from build123d import *
from OCP.BRepFilletAPI import BRepFilletAPI_MakeChamfer

# Parameters (mm, degrees)
BOSS_EXTRUDE1_DEPTH = 30
CUT_EXTRUDE1_REACH  = 253.063
SKETCH10_W          = 41.5
SKETCH10_H          = 34
BOSS_EXTRUDE3_DEPTH = 4
CHAMFER4_SIZE       = 20
CHAMFER4_SIZE2      = 11.547005384
SKETCH11_W          = 20.75
SKETCH11_H          = 166.64
BOSS_EXTRUDE4_DEPTH = 4
SKETCH12_W          = 20.75
SKETCH12_H          = 18.32
BOSS_EXTRUDE5_DEPTH = 4
SKETCH13_W          = 75
SKETCH13_H          = 20
SKETCH13_W_2        = 20
SKETCH13_H_2        = 90
CUT_EXTRUDE2_DEPTH  = 4
FILLET1_R           = 3
CUT_EXTRUDE3_REACH  = 188.866
SKETCH15_R          = 1.6
CUT_EXTRUDE4_START  = -2
SKETCH16_R          = 3.5
SKETCH16_R_2        = 1.6
CUT_EXTRUDE4_DEPTH  = 2


with BuildPart() as part:
    # Sketch6 → Boss-Extrude1 (new body)
    with BuildSketch(Plane(origin=(0, 0, 0), x_dir=(1, 0, 0), z_dir=(0, 1, 0))):
        Polygon((0, -87.32), (37.5, -87.32), (37.5, -117.32), (90.67, -117.32), (142.319755082, -87.5), (142.319755082, 87.5), (90.67, 117.32), (37.5, 117.32), (37.5, 87.32), (0, 87.32), (0, 83.32), (41.5, 83.32), (41.5, 113.32), (89.59820323, 113.32), (138.319755082, 85.190598923), (138.319755082, -85.190598923), (89.59820323, -113.32), (41.5, -113.32), (41.5, -83.32), (0, -83.32), align=None)
    extrude(amount=BOSS_EXTRUDE1_DEPTH)

    # Sketch9 → Cut-Extrude1 (cut, up to next)
    with BuildSketch(Plane.XY.offset(87.32), mode=Mode.PRIVATE) as cut_extrude1_sk1:
        Polygon((37.5, 0), (15, 8), (0, 8), (0, 0), align=None)
    cut_extrude1_tool1 = extrude(cut_extrude1_sk1.sketch, amount=-CUT_EXTRUDE1_REACH, mode=Mode.PRIVATE) & part.part
    cut_extrude1 = cut_extrude1_tool1.solids().sort_by_distance((13.928571, 3.428571, 87.32))[0]
    add(cut_extrude1, mode=Mode.SUBTRACT)

    # Sketch10 → Boss-Extrude3 (add)
    with BuildSketch(Plane(origin=(0, 30, 0), x_dir=(1, 0, 0), z_dir=(0, 1, 0))):
        with Locations((20.75, -100.32)):
            Rectangle(SKETCH10_W, SKETCH10_H)
    boss_extrude3 = extrude(amount=-BOSS_EXTRUDE3_DEPTH)

    # Mirror1: Cut-Extrude1, Boss-Extrude3 across plane
    add(cut_extrude1.mirror(Plane.XY), mode=Mode.SUBTRACT)
    add(boss_extrude3.mirror(Plane.XY))

    # Chamfer4: one chamfer whose edges measure the first distance from different faces: ONE call of the kernel's chamfer builder (chamfer() names one face for all edges)
    chamfer4_edges_1 = [part.edges().sort_by_distance(p)[0] for p in [
        (37.5, 26, -102.32),
    ]]
    chamfer4_side_1 = [part.faces().sort_by_distance(p)[0] for p in [
        (18.75, 26, -102.32),
    ]]
    chamfer4_edges_2 = [part.edges().sort_by_distance(p)[0] for p in [
        (37.5, 26, 102.32),
    ]]
    chamfer4_side_2 = [part.faces().sort_by_distance(p)[0] for p in [
        (18.75, 26, 102.32),
    ]]
    chamfer4 = BRepFilletAPI_MakeChamfer(part.part.solid().wrapped)
    for e in chamfer4_edges_1:
        chamfer4.Add(CHAMFER4_SIZE, CHAMFER4_SIZE2, e.wrapped, chamfer4_side_1[0].wrapped)  # the first distance lies on this face
    for e in chamfer4_edges_2:
        chamfer4.Add(CHAMFER4_SIZE, CHAMFER4_SIZE2, e.wrapped, chamfer4_side_2[0].wrapped)  # the first distance lies on this face
    add(Compound.cast(chamfer4.Shape()), mode=Mode.REPLACE)

    # Sketch11 → Boss-Extrude4 (add)
    with BuildSketch(Plane(origin=(0, 30, 0), x_dir=(1, 0, 0), z_dir=(0, 1, 0))):
        with Locations((10.375, 0)):
            Rectangle(SKETCH11_W, SKETCH11_H)
    extrude(amount=-BOSS_EXTRUDE4_DEPTH)

    # Sketch12 → Boss-Extrude5 (add)
    with BuildSketch(Plane(origin=(0, 30, 0), x_dir=(1, 0, 0), z_dir=(0, 1, 0))):
        Polygon((41.5, 65), (20.75, 65), (20.75, -65), (41.5, -65), (138.319755082, -65), (138.319755082, 65), align=None)
        with Locations((31.125, -74.16)):
            Rectangle(SKETCH12_W, SKETCH12_H)
        with Locations((31.125, 74.16)):
            Rectangle(SKETCH12_W, SKETCH12_H)
    extrude(amount=-BOSS_EXTRUDE5_DEPTH)

    # Sketch13 → Cut-Extrude2 (cut)
    with BuildSketch(Plane(origin=(0, 30, 0), x_dir=(1, 0, 0), z_dir=(0, 1, 0))):
        with Locations((89.909877541, 35)):
            Rectangle(SKETCH13_W, SKETCH13_H)
        with Locations((89.909877541, 0)):
            Rectangle(SKETCH13_W, SKETCH13_H)
        with Locations((89.909877541, -35)):
            Rectangle(SKETCH13_W, SKETCH13_H)
        with Locations((27.409877541, 0)):
            Rectangle(SKETCH13_W_2, SKETCH13_H_2)
    extrude(amount=-CUT_EXTRUDE2_DEPTH, mode=Mode.SUBTRACT)

    # Fillet1
    fillet1_edges = [part.edges().sort_by_distance(p)[0] for p in [
        (37.409877541, 28, -45),
        (37.409877541, 28, 45),
        (17.409877541, 28, 45),
        (17.409877541, 28, -45),
        (52.409877541, 28, 45),
        (52.409877541, 28, 25),
        (127.409877541, 28, 25),
        (127.409877541, 28, 45),
        (52.409877541, 28, 10),
        (52.409877541, 28, -10),
        (127.409877541, 28, -10),
        (127.409877541, 28, 10),
        (52.409877541, 28, -25),
        (52.409877541, 28, -45),
        (127.409877541, 28, -45),
        (127.409877541, 28, -25),
    ]]
    fillet(fillet1_edges, radius=FILLET1_R)

    # Sketch15 → Cut-Extrude3 (cut, up to next)
    with BuildSketch(Plane(origin=(0, 30, 0), x_dir=(1, 0, 0), z_dir=(0, 1, 0)), mode=Mode.PRIVATE) as cut_extrude3_sk1:
        with Locations(Location((111, 61, 0), (0, 0, 270))):
            Circle(SKETCH15_R)
    cut_extrude3_tool1 = extrude(cut_extrude3_sk1.sketch, amount=-CUT_EXTRUDE3_REACH, mode=Mode.PRIVATE) & part.part
    # Sketch15 → Cut-Extrude3 (cut, up to next)
    with BuildSketch(Plane(origin=(0, 30, 0), x_dir=(1, 0, 0), z_dir=(0, 1, 0)), mode=Mode.PRIVATE) as cut_extrude3_sk2:
        with Locations(Location((111, -61, 0), (0, 0, 270))):
            Circle(SKETCH15_R)
    cut_extrude3_tool2 = extrude(cut_extrude3_sk2.sketch, amount=-CUT_EXTRUDE3_REACH, mode=Mode.PRIVATE) & part.part
    # Sketch15 → Cut-Extrude3 (cut, up to next)
    with BuildSketch(Plane(origin=(0, 30, 0), x_dir=(1, 0, 0), z_dir=(0, 1, 0)), mode=Mode.PRIVATE) as cut_extrude3_sk3:
        with Locations(Location((24, -61, 0), (0, 0, 270))):
            Circle(SKETCH15_R)
    cut_extrude3_tool3 = extrude(cut_extrude3_sk3.sketch, amount=-CUT_EXTRUDE3_REACH, mode=Mode.PRIVATE) & part.part
    # Sketch15 → Cut-Extrude3 (cut, up to next)
    with BuildSketch(Plane(origin=(0, 30, 0), x_dir=(1, 0, 0), z_dir=(0, 1, 0)), mode=Mode.PRIVATE) as cut_extrude3_sk4:
        with Locations(Location((24, 61, 0), (0, 0, 270))):
            Circle(SKETCH15_R)
    cut_extrude3_tool4 = extrude(cut_extrude3_sk4.sketch, amount=-CUT_EXTRUDE3_REACH, mode=Mode.PRIVATE) & part.part
    add(cut_extrude3_tool1.solids().sort_by_distance((111, 30, -61))[0], mode=Mode.SUBTRACT)
    add(cut_extrude3_tool2.solids().sort_by_distance((111, 30, 61))[0], mode=Mode.SUBTRACT)
    add(cut_extrude3_tool3.solids().sort_by_distance((24, 30, 61))[0], mode=Mode.SUBTRACT)
    add(cut_extrude3_tool4.solids().sort_by_distance((24, 30, -61))[0], mode=Mode.SUBTRACT)

    # Sketch16 → Cut-Extrude4 (cut)
    # profile 1 of 12: a face of its own
    with BuildSketch(Plane.XZ.offset(-26).offset(CUT_EXTRUDE4_START)):
        with Locations(Location((24, 61, 0), (0, 0, 270))):
            Circle(SKETCH16_R)
        with Locations(Location((24, 61, 0), (0, 0, 90))):
            Circle(SKETCH16_R_2, mode=Mode.SUBTRACT)
    # profile 2 of 12: a face of its own
    with BuildSketch(Plane.XZ.offset(-26).offset(CUT_EXTRUDE4_START)):
        with BuildLine():
            ThreePointArc((109.4, 61), (111, 62.6), (112.6, 61))
            Line((112.6, 61), (114.5, 61))
            ThreePointArc((114.5, 61), (111, 64.5), (107.5, 61))
            Line((107.5, 61), (109.4, 61))
        make_face()
    # profile 3 of 12: a face of its own
    with BuildSketch(Plane.XZ.offset(-26).offset(CUT_EXTRUDE4_START)):
        with BuildLine():
            Line((114.5, 61), (112.6, 61))
            ThreePointArc((112.6, 61), (111, 59.4), (109.4, 61))
            Line((109.4, 61), (107.5, 61))
            ThreePointArc((107.5, 61), (111, 57.5), (114.5, 61))
        make_face()
    # profile 4 of 12: a face of its own
    with BuildSketch(Plane.XZ.offset(-26).offset(CUT_EXTRUDE4_START)):
        with BuildLine():
            ThreePointArc((109.4, 61), (111, 62.6), (112.6, 61))
            Line((112.6, 61), (114.5, 61))
            ThreePointArc((114.5, 61), (111, 64.5), (107.5, 61))
            Line((107.5, 61), (109.4, 61))
        make_face()
    # profile 5 of 12: a face of its own
    with BuildSketch(Plane.XZ.offset(-26).offset(CUT_EXTRUDE4_START)):
        with BuildLine():
            Line((114.5, 61), (112.6, 61))
            ThreePointArc((112.6, 61), (111, 59.4), (109.4, 61))
            Line((109.4, 61), (107.5, 61))
            ThreePointArc((107.5, 61), (111, 57.5), (114.5, 61))
        make_face()
    # profile 6 of 12: a face of its own
    with BuildSketch(Plane.XZ.offset(-26).offset(CUT_EXTRUDE4_START)):
        with BuildLine():
            ThreePointArc((107.5, 61), (111, 64.5), (114.5, 61))
            Line((114.5, 61), (114.5, 65))
            Line((114.5, 65), (107.5, 65))
            Line((107.5, 65), (107.5, 61))
        make_face()
    # profile 7 of 12: a face of its own
    with BuildSketch(Plane.XZ.offset(-26).offset(CUT_EXTRUDE4_START)):
        with BuildLine():
            Line((114.5, -65), (114.5, -61))
            ThreePointArc((114.5, -61), (111, -64.5), (107.5, -61))
            Line((107.5, -61), (107.5, -65))
            Line((107.5, -65), (114.5, -65))
        make_face()
    # profile 8 of 12: a face of its own
    with BuildSketch(Plane.XZ.offset(-26).offset(CUT_EXTRUDE4_START)):
        with BuildLine():
            ThreePointArc((109.4, -61), (111, -59.4), (112.6, -61))
            Line((112.6, -61), (114.5, -61))
            ThreePointArc((114.5, -61), (111, -57.5), (107.5, -61))
            Line((107.5, -61), (109.4, -61))
        make_face()
    # profile 9 of 12: a face of its own
    with BuildSketch(Plane.XZ.offset(-26).offset(CUT_EXTRUDE4_START)):
        with BuildLine():
            Line((114.5, -61), (112.6, -61))
            ThreePointArc((112.6, -61), (111, -62.6), (109.4, -61))
            Line((109.4, -61), (107.5, -61))
            ThreePointArc((107.5, -61), (111, -64.5), (114.5, -61))
        make_face()
    # profile 10 of 12: a face of its own
    with BuildSketch(Plane.XZ.offset(-26).offset(CUT_EXTRUDE4_START)):
        with BuildLine():
            ThreePointArc((109.4, -61), (111, -59.4), (112.6, -61))
            Line((112.6, -61), (114.5, -61))
            ThreePointArc((114.5, -61), (111, -57.5), (107.5, -61))
            Line((107.5, -61), (109.4, -61))
        make_face()
    # profile 11 of 12: a face of its own
    with BuildSketch(Plane.XZ.offset(-26).offset(CUT_EXTRUDE4_START)):
        with BuildLine():
            Line((114.5, -61), (112.6, -61))
            ThreePointArc((112.6, -61), (111, -62.6), (109.4, -61))
            Line((109.4, -61), (107.5, -61))
            ThreePointArc((107.5, -61), (111, -64.5), (114.5, -61))
        make_face()
    # profile 12 of 12: a face of its own
    with BuildSketch(Plane.XZ.offset(-26).offset(CUT_EXTRUDE4_START)):
        with Locations(Location((24, -61, 0), (0, 0, 270))):
            Circle(SKETCH16_R)
        with Locations(Location((24, -61, 0), (0, 0, 90))):
            Circle(SKETCH16_R_2, mode=Mode.SUBTRACT)
    extrude(amount=CUT_EXTRUDE4_DEPTH, mode=Mode.SUBTRACT)


solid = part.part
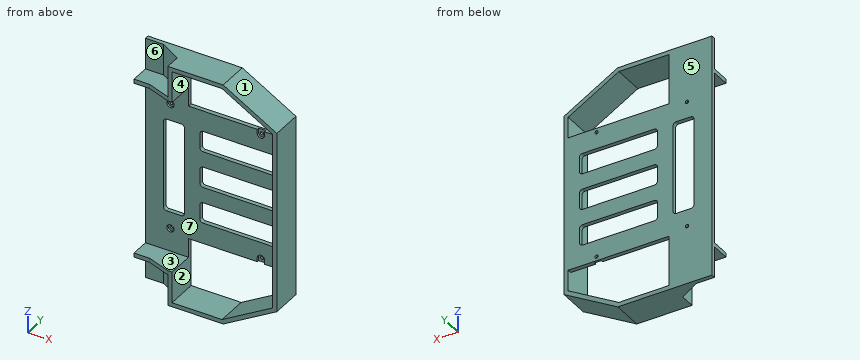
The listing builds one solid part. Answer for the finished solid, in the listing's coordinates (mm). Face numbers are marked on the shaded views. A direction names the side the tool comes from. Give positions to 0.01 mm unless a question says otherwise; leave off trailing zeros. Write each loop counter-clockwise with the first axis right and the second up, starting at its lowest first coordinate (ties: lowest second). Pieces come first, ordered by that corner, then holes.
1) Section D-D (x = 76.5) is taken. Write down the section's boundary in (y, z), and give its area (3 significant figures).
2) Given P1, Ø3, axis at x = 104.5, y = 29, coming from the +Z side; P2, Ø4.5, axis at x = 105, y = 29, coming from the -Z side; P3, Ø9, axis at y = 13.5, z = -29.5, coming from the -X side, each flat-ended and moving along its own axis, determine where each tip first touches the part or whether it passes through.
3) Find the intervals of material crossed by L1, parallel to X at y = 28.7, z = 61; L2, parallel to X at y = 28, z = 42.5; L3, parallel to Z at x = 24, y = 29.35, in increasing order.
4) Section A-A (x = 50) is taken. Write down the section's boundary in (y, z).
5) For a pull along X with two mould halves and no side action, classify the marked faces 1, 2 and 3 as pulls with the +X half, pulls with the -X half, needs draft (parallel to the pull), parting line crosses it, or undercut.
6) Section B-B (z = 30.5) is taken. Write down the section's boundary in (x, y), and give its area (3 significant figures).
7) A tool of negligible diameter and unlimited length cuts with its end or side. For the marked faces 4, 5, 6 and 7, from which of +Z, -Z, +X, -X, +Y, -Y can it reach the whole face along a straight path? Write none if from no direction.
8) Section C-C (z = -80) is taken. Write down the section's boundary in (x, y), and give its area (3 significant figures).
Response:
1. outline: (0, -117.32) - (30, -117.32) - (30, -113.32) - (0, -113.32) - close; (0, 113.32) - (30, 113.32) - (30, 117.32) - (0, 117.32) - close; (26, -65) - (30, -65) - (30, -45) - (26, -45) - close; (26, -25) - (30, -25) - (30, -10) - (26, -10) - close; (26, 10) - (30, 10) - (30, 25) - (26, 25) - close; (26, 45) - (30, 45) - (30, 65) - (26, 65) - close
1. area: 520 mm2
2. P1: stops at z = 110.2
2. P2: stops at z = -110.35
2. P3: stops at x = 138.32
3. L1: x = 0 to 22.4, 25.6 to 109.4, 112.6 to 142.32
3. L2: x = 0 to 17.45, 37.37 to 52.45, 127.37 to 142.32
3. L3: z = -117.32 to -62.6, -59.4 to -45, 45 to 59.4, 62.6 to 117.32
4. outline: (0, -117.32) - (30, -117.32) - (30, -113.32) - (0, -113.32) - close; (0, 113.32) - (30, 113.32) - (30, 117.32) - (0, 117.32) - close; (26, -65) - (30, -65) - (30, 65) - (26, 65) - close
5. face 1: pulls with the +X half
5. face 2: undercut
5. face 3: needs draft
6. outline: (0, 26) - (17.41, 26) - (17.41, 30) - (0, 30) - close; (37.41, 26) - (52.41, 26) - (52.41, 30) - (37.41, 30) - close; (127.41, 26) - (138.32, 26) - (138.32, 0) - (142.32, 0) - (142.32, 30) - (127.41, 30) - close
6. area: 293 mm2
7. face 4: +Y, -Y
7. face 5: +Z, -Z, +X, -X, +Y
7. face 6: +Z, -X, -Y
7. face 7: -X, -Y
8. outline: (0, 26) - (41.5, 26) - (41.5, 30) - (0, 30) - close; (138.32, 0) - (142.32, 0) - (142.32, 30) - (138.32, 30) - close
8. area: 286 mm2
